```python
from build123d import *

# Parameters (mm, degrees)
SKETCH1_W           = 18.796
SKETCH1_H           = 18.796
BOSS_EXTRUDE1_DEPTH = 3.048
SKETCH3_W           = 18.796
SKETCH3_H           = 18.796
BOSS_EXTRUDE2_DEPTH = 3.048
SKETCH4_W           = 15.24
SKETCH4_H           = 15.24
CUT_EXTRUDE1_DEPTH  = 1.651
SKETCH5_W           = 15.24
SKETCH5_H           = 15.24
CUT_EXTRUDE2_DEPTH  = 1.651
SKETCH6_W           = 2.54
SKETCH6_H           = 1.524
SKETCH6_W_2         = 1.524
SKETCH6_H_2         = 2.54
CUT_EXTRUDE3_DEPTH  = 1.651
SKETCH7_W           = 2.54
SKETCH7_H           = 1.524
SKETCH7_W_2         = 1.524
SKETCH7_H_2         = 2.54
CUT_EXTRUDE4_DEPTH  = 24.020304603
BOSS_EXTRUDE3_DEPTH = 1.651
FILLET1_R           = 0.508
FILLET2_R           = 0.508


with BuildPart() as part:
    # Sketch1 → Boss-Extrude1 (new body)
    with BuildSketch(Plane.XY):
        Rectangle(SKETCH1_W, SKETCH1_H)
    extrude(amount=-BOSS_EXTRUDE1_DEPTH)

    # Sketch3 → Boss-Extrude2 (add)
    with BuildSketch(Plane(origin=(0, 9.398, 0), x_dir=(1, 0, 0), z_dir=(0, 1, 0))):
        with Locations((0, 9.398)):
            Rectangle(SKETCH3_W, SKETCH3_H)
    extrude(amount=-BOSS_EXTRUDE2_DEPTH)

    # Sketch4 → Cut-Extrude1 (cut)
    with BuildSketch(Plane(origin=(0, 9.398, 0), x_dir=(1, 0, 0), z_dir=(0, 1, 0))):
        with Locations((0, 9.398)):
            Rectangle(SKETCH4_W, SKETCH4_H)
    extrude(amount=-CUT_EXTRUDE1_DEPTH, mode=Mode.SUBTRACT)

    # Sketch5 → Cut-Extrude2 (cut)
    with BuildSketch(Plane.XY):
        Rectangle(SKETCH5_W, SKETCH5_H)
    extrude(amount=-CUT_EXTRUDE2_DEPTH, mode=Mode.SUBTRACT)

    # Sketch6 → Cut-Extrude3 (cut)
    with BuildSketch(Plane(origin=(0, 7.747, 0), x_dir=(1, 0, 0), z_dir=(0, 1, 0))):
        with Locations((0, 5.20193254)):
            Rectangle(SKETCH6_W, SKETCH6_H)
        with Locations((-4.064, 9.26593254)):
            Rectangle(SKETCH6_W_2, SKETCH6_H_2)
        with Locations((4.064, 9.26593254)):
            Rectangle(SKETCH6_W_2, SKETCH6_H_2)
        with Locations((0, 13.32993254)):
            Rectangle(SKETCH6_W, SKETCH6_H)
    extrude(amount=-CUT_EXTRUDE3_DEPTH, mode=Mode.SUBTRACT)

    # Sketch7 → Cut-Extrude4 (cut, through all)
    with BuildSketch(Plane.XY):
        with Locations((0, 4.064)):
            Rectangle(SKETCH7_W, SKETCH7_H)
        with Locations((4.064, 0)):
            Rectangle(SKETCH7_W_2, SKETCH7_H_2)
        with Locations((0, -4.064)):
            Rectangle(SKETCH7_W, SKETCH7_H)
        with Locations((-4.064, 0)):
            Rectangle(SKETCH7_W_2, SKETCH7_H_2)
    extrude(amount=-CUT_EXTRUDE4_DEPTH, mode=Mode.SUBTRACT)

    # Sketch8 → Boss-Extrude3 (add)
    with BuildSketch(Plane(origin=(9.398, 0, 0), x_dir=(0, 0, -1), z_dir=(1, 0, 0))):
        Polygon((3.048, 6.35), (3.048, -8.89), (6.096, -8.89), (7.366, -7.62), (7.874, -7.62), (17.526, 2.032), (17.526, 2.54), (18.288, 3.302), (18.288, 6.35), align=None)
    extrude(amount=-BOSS_EXTRUDE3_DEPTH)

    # Fillet1
    fillet1_edges = [part.edges().sort_by_distance(p)[0] for p in [
        (7.62, 8.5725, -1.778),
        (-7.62, 8.5725, -1.778),
        (-7.62, 8.5725, -17.018),
        (7.62, 8.5725, -17.018),
    ]]
    fillet(fillet1_edges, radius=FILLET1_R)

    # Fillet2
    fillet2_edges = [part.edges().sort_by_distance(p)[0] for p in [
        (-7.62, -7.62, -0.8255),
        (-7.62, 7.62, -0.8255),
        (7.62, 7.62, -0.8255),
        (7.62, -7.62, -0.8255),
    ]]
    fillet(fillet2_edges, radius=FILLET2_R)


solid = part.part
```
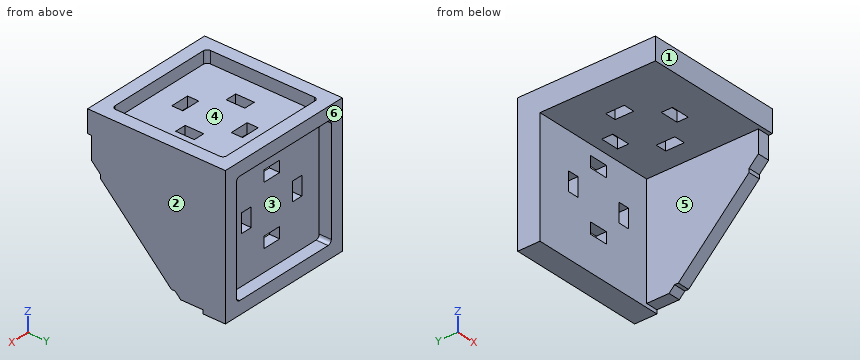
For this review, take the finished solid that the model builds, in its own axes (mm). Face numbers are marked on the shaded views. A direction names the side the tool comes from. Give positions to 0.01 mm unless a question says otherwise; leave off trailing zeros. Write each loop counter-clockwise with the first axis right and the second up, starting at its lowest first coordinate (ties: lowest second). Pieces come first, ordered by that corner, then holes. Notation, with made-up numbers: M -36,8.5 L 14,8.5 A25 cw 14,35.5 Z; hole C -16,-31 d6. An arc over 180 degrees is marked long. Answer as a JSON object with one key per item and string values. Group by question number.
Item 1: For pin 1 Ø3 at (x, y) = (7, 1) entering from -Z; pin 2 Ø2 at (y, z) = (-2.5, -7.5) entering from -X; pin 3 Ø3 at (x, z) = (-5, -7) entering from -Y, all flat-tipped, find the tip position at first contact; note any pin that passes through.
Item 2: Consider section B-B on y = 4. Write out the cut boundary in (x, z).
Item 3: Draft analysis for pull direction X (two halves, no side actions). For the marked faces 1, 2 and 3, state which applies: +X half, -X half, draft (parallel to the pull), parting line (faces both ways), or undercut.
Item 4: For probe 1 along Y at (x, z) = (-6.25, -1.25); probe 2 along Z at (x, y) = (-4, 7), list the stretches that pass through material, from the lowest coordinate up. Write a range as [from, to].
Item 5: Consider section C-C on x = -0.75. Count the separate pieces of the cut face and the enclosed holes in it, plus the area to 3 significant figures.
Item 6: Consider section A-A on z = -5.5. Write out the cut boundary in (x, y), plus the area to 3 significant figures.
Item 7: Tool access review of the marked faces 4, 5 and 6: name each direction out of +Z, -Z, +X, -X, +Y, -Y from which nothing blocks a thin tool from reaching the whole face with its end or side.
Item 8: Consider section D-D on z = -2.75. Write out the cut boundary in (x, y).
Check result:
{
 "1": {"pin 1": "stops at z = -17.53", "pin 2": "stops at x = 7.75", "pin 3": "stops at y = 6.35"},
 "2": {"outline": "M -9.4,-3.05 L -1.27,-3.05 L -1.27,-1.65 L -7.62,-1.65 L -7.62,0 L -9.4,0 Z; M 1.27,-3.05 L 7.75,-3.05 L 7.75,-18.29 L 9.4,-18.29 L 9.4,0 L 7.62,0 L 7.62,-1.65 L 1.27,-1.65 Z"},
 "3": {"face 1": "draft", "face 2": "+X half", "face 3": "undercut"},
 "4": {"probe 1": "y = [-9.4, -7.62], [7.62, 9.4]", "probe 2": "z = [-18.8, -10.54], [-8, -1.65]"},
 "5": {"separate pieces": "5", "enclosed holes": "0", "area": "46.5 mm^2"},
 "6": {"outline": "M -9.4,6.35 L -1.27,6.35 L -1.27,7.75 L -7.62,7.75 L -7.62,9.4 L -9.4,9.4 Z; M 1.27,6.35 L 7.75,6.35 L 7.75,-8.89 L 9.4,-8.89 L 9.4,9.4 L 7.62,9.4 L 7.62,7.75 L 1.27,7.75 Z", "area": "53.7 mm^2"},
 "7": {"face 4": "+Z", "face 5": "-Z, -X, -Y", "face 6": "+Z, -Z, +X, -X, +Y"},
 "8": {"outline": "M -9.4,-9.4 L 9.4,-9.4 L 9.4,9.4 L 7.62,9.4 L 7.62,7.75 L -7.62,7.75 L -7.62,9.4 L -9.4,9.4 Z; hole M -4.83,-1.27 L -3.3,-1.27 L -3.3,1.27 L -4.83,1.27 Z; hole M -1.27,-4.83 L 1.27,-4.83 L 1.27,-3.3 L -1.27,-3.3 Z; hole M -1.27,3.3 L 1.27,3.3 L 1.27,4.83 L -1.27,4.83 Z; hole M 3.3,-1.27 L 4.83,-1.27 L 4.83,1.27 L 3.3,1.27 Z"}
}
